CAD build for the part. Positions are in the model's coordinates, mm. Coordinates: 2 decimals unless noted, no trailing zeros. Loops run counter-clockwise (first coordinate to the right, second up) from the corner with the lowest first, then second, coordinate; pieces in that order, holes last. Notation, with made-up numbers: (23.5, -8) -> (70.5, -8) arc R30 ccw to (70.5, 25) -> close; hole circle Ø3 at (71, 9.5). An arc over 180 degrees is marked (long way). Return JSON: item names as keys, results as strings. Group by question number.
(1) Saw through at A-A on y = 5. Write the cut outline in (x, z), then the cut area to 3 significant figures.
(2) Saw through at B-B on z = 32. Write the cut outline in (x, y).
(3) Flat gauge pins, fed straight in: pin 1 Ø10 at (y, z) = (35, 16) entering from -X; pin 2 Ø5 at (x, y) = (8, 17) entering from +Z; pin 3 Ø4 at (y, z) = (20.5, 33.5) entering from +X; pin 4 Ø10 at (x, y) = (21, 35.5) entering from +Z. Where does each tip first touch, or does it go through?
(4) Saw through at D-D on y = 19. Write the cut outline in (x, z), then the cut area to 3 significant figures.
(5) Probe L1, parallel to Z at x = 23.5, y = 37.5; L2, parallel to X at y = 4.5, z = 9; L3, parallel to X at y = 15.5, z = 38.5. List the from-to ranges inside material, lowest first.
(6) Saw through at C-C on x = 5. Write the cut outline in (y, z).
```python
from build123d import *

# Parameters (mm, degrees)
SKETCH1_W           = 40
SKETCH1_H           = 40
BOSS_EXTRUDE1_DEPTH = 40
CUT_EXTRUDE1_DEPTH  = 40
CUT_EXTRUDE2_DEPTH  = 40


with BuildPart() as part:
    # Sketch1 → Boss-Extrude1 (new body)
    with BuildSketch(Plane.XY):
        with Locations((20, 20)):
            Rectangle(SKETCH1_W, SKETCH1_H)
    extrude(amount=BOSS_EXTRUDE1_DEPTH)

    # Sketch2 → Cut-Extrude1 (cut)
    with BuildSketch(Plane.XY.offset(40)):
        Polygon((0, 0), (20, 40), (0, 40), align=None)
    extrude(amount=-CUT_EXTRUDE1_DEPTH, mode=Mode.SUBTRACT)

    # Sketch3 → Cut-Extrude2 (cut)
    with BuildSketch(Plane.XZ):
        Polygon((0, 40), (0, 30), (20, 40), align=None)
        Polygon((0, 0), (20, 0), (0, 10), align=None)
        Polygon((20, 40), (40, 30), (40, 40), align=None)
        Polygon((40, 10), (20, 0), (40, 0), align=None)
    extrude(amount=-CUT_EXTRUDE2_DEPTH, mode=Mode.SUBTRACT)


solid = part.part
```
Geometry results:
{
 "1": {"outline": "(2.5, 8.75) -> (20, 0) -> (40, 10) -> (40, 30) -> (20, 40) -> (2.5, 31.25) -> close", "area": "1,150 mm²"},
 "2": {"outline": "(4, 0) -> (36, 0) -> (36, 40) -> (20, 40) -> (4, 8) -> close"},
 "3": {"pin 1": "x = 15", "pin 2": "z = 35.25", "pin 3": "x = 37", "pin 4": "z = 40"},
 "4": {"outline": "(9.5, 5.25) -> (20, 0) -> (40, 10) -> (40, 30) -> (20, 40) -> (9.5, 34.75) -> close", "area": "965 mm²"},
 "5": {"L1": "1.75 to 38.25", "L2": "2.25 to 38", "L3": "17 to 23"},
 "6": {"outline": "(0, 7.5) -> (10, 7.5) -> (10, 32.5) -> (0, 32.5) -> close"}
}
